Read the model definition and answer for the solid it produces. Units are mm, in the model's axes. A direction names the side the tool comes from. Give positions to 0.01 mm unless a question says otherwise; leave off trailing zeros. Order: outer loops, then holes, each group sorted by start corner. A loop starts at its lowest first (then second) coordinate and runs counter-clockwise, first axis right, second up. Notation, with made-up numbers: (-28.5, 89.5) - (-3.5, 89.5) arc R34 ccw to (-3.5, 122.5) - close; hole circle Ø1 at (86, -17.5). An arc over 180 degrees is marked (long way). Write each question's results on one line, items separated by ' | '.
Autodesk Inventor part; units mm, degrees
ref_plane "YZ Plane" through (0, 0, 0) normal (1, 0, 0) x (0, 1, 0)
ref_plane "XZ Plane" through (0, 0, 0) normal (0, 1, 0) x (-1, 0, 0)
ref_plane "XY Plane" through (0, 0, 0) normal (0, 0, 1) x (1, 0, 0)
sketch "Sketch2" plane through (0, 0, 0) normal (0, 0, 1) x (1, 0, 0)
  line L0 (0, 4) -> (0.5, 4.5)
  line L1 (0, 4) -> (0, 3)
  line L2 (0.5, 4.5) -> (1.1, 4.5)
  line L3 (1.1, 4.5) -> (1.1, 4.3)
  line L4 (1.1, 4.3) -> (2.1, 4.3)
  line L5 (2.1, 4.3) -> (2.1, 4.5)
  line L6 (2.1, 4.5) -> (14.8, 4.5)
  line L7 (15.1, 4.5) -> (15.1, 5.5)
  line L8 (15.1, 5.5) -> (15.6, 6)
  line L9 (44.15, 4.5) -> (44.15, 4.3)
  line L10 (44.15, 4.3) -> (43.15, 4.3)
  line L11 (43.15, 4.3) -> (43.15, 4.5)
  line L12 (0, 0) -> (27.0854, 0) construction
  line L13 (15.6, 6) -> (16.1, 6)
  line L14 (16.1, 6) -> (16.1, 5)
  line L15 (16.1, 5) -> (17.1, 5)
  line L16 (17.1, 5) -> (17.1, 6)
  line L17 (31.9, 6) -> (31.8, 6)
  line L18 (31.5, 6) -> (31.5, 6.5)
  line L19 (31.5, 6.5) -> (28.1, 6.5)
  line L20 (28.1, 6.5) -> (28.1, 6)
  line L21 (17.1, 6) -> (28.1, 6)
  line L22 (21, 3.2) -> (43.9, 3.2)
  line L23 (44.15, 4.5) -> (45.15, 4.5)
  line L24 (43.15, 4.5) -> (37.9, 4.5)
  line L25 (37.15, 6) -> (31.9, 6)
  line L26 (43.9, 3.2) -> (49.9, 3.2)
  line L27 (49.9, 4) -> (45.45, 4)
  line L28 (45.15, 4) -> (45.15, 4.5)
  line L29 (49.9, 3.2) -> (51.9, 3.2)
  line L30 (51.9, 3.2) -> (51.9, 4)
  line L31 (51.9, 4) -> (49.9, 4)
  line L32 (37.9, 4.5) -> (37.45, 4.5)
  line L33 (37.15, 4.5) -> (37.15, 6)
  line L34 (15.1, 4.5) -> (15.1, 4.3)
  line L35 (15.1, 4.3) -> (14.8, 4.3)
  line L36 (14.8, 4.3) -> (14.8, 4.5)
  line L37 (31.5, 6) -> (31.5, 5.8)
  line L38 (31.5, 5.8) -> (31.8, 5.8)
  line L39 (31.8, 5.8) -> (31.8, 6)
  line L40 (37.15, 4.5) -> (37.15, 4.3)
  line L41 (37.15, 4.3) -> (37.45, 4.3)
  line L42 (37.45, 4.3) -> (37.45, 4.5)
  line L43 (45.15, 4) -> (45.15, 3.8)
  line L44 (45.15, 3.8) -> (45.45, 3.8)
  line L45 (45.45, 3.8) -> (45.45, 4)
  line L46 (0, 3) -> (0, 0)
  line L47 (0, 0) -> (20, 0)
  line L48 (20, 2.2) -> (20, 0)
  line L49 (20, 2.2) -> (21, 3.2)
  point P0 (1.1, 4.4)
  point P1 (15.85, 6)
  point P2 (16.6, 5)
  dimension "d3" = 4
  dimension "d8" = 1
  dimension "d9" = 0.5
  dimension "d10" = 0.5
  dimension "d11" = 0.2
  dimension "d12" = 1
  dimension "d13" = 13
  dimension "d14" = 1
  dimension "d29" = 0.5
  dimension "d30" = 0.5
  dimension "d36" = 1.1
  dimension "d37" = 4.5
  dimension "d38" = 3
  dimension "d39" = 0.5
  dimension "d40" = 1
  dimension "d41" = 1
  dimension "d60" = 0.4
  dimension "d61" = 0.5
  dimension "d62" = 3.4
  dimension "d63" = 11
  dimension "d65" = 1
  dimension "d66" = 5.25
  dimension "d83" = 6
  dimension "d84" = 0.8
  dimension "d85" = 2
  dimension "d86" = 0.75
  dimension "d105" = 0.2
  dimension "d106" = 0.3
  dimension "d107" = 0.2
  dimension "d108" = 0.3
  dimension "d109" = 0.2
  dimension "d110" = 0.3
  dimension "d111" = 0.2
  dimension "d112" = 0.3
revolve "Revolution1" add sketch "Sketch2" angle 360 about axis through (0, 0, 0) along (1, 0, 0)
thread "Thread1"
ref_plane "Work Plane1" through (51.1424, -20, -139.2633) normal (0, 1, 0) x (-1, 0, 0)
sketch "Sketch4" plane through (17.1, 0, 0) normal (-1, 0, 0) x (0, 0, 1)
  circle A0 centre (0, 0) radius 6
  point P0 (0, 6)
  point P1 (6, 0)
  point P2 (0, -6.0107)
  point P3 (-6.0435, 0)
chamfer "Chamfer3" distance 0.3 angle 45 1 edges at (51.9, -4, 0)
ref_plane "Work Plane4" through (17.1, 0, 6) normal (0, 0, 1) x (1, 0, 0)
sketch "Sketch8" plane through (17.1, 0, 6) normal (0, 0, 1) x (1, 0, 0)
  circle A0 centre (6.1, 0) radius 1
  line L0 (0, -6) -> (0, 6)
  point P0 (-17.1, 0)
  dimension "d90" = 2
  dimension "d91" = 6.1
hole "Hole3" at (23.2, 0, 6) direction (0, 0, -1) diameter 1.567 depth 6.3 tip angle 118
chamfer "Chamfer4" distance 0.2 angle 45 3 edges at (22.6668, -0.5741, 5.9725) (23.7332, -0.5741, 5.9725) (23.2, 0.7835, 5.9486)
chamfer "Chamfer5" distance 0.3 angle 45 1 edges at (51.9, -3.2, 0)
sketch "Sketch9" plane through (0, 0, 0) normal (-1, 0, 0) x (0, 0, 1)
  circle A0 centre (0, 0) radius 1.2953
hole "Hole4" at (0, 0, 0) direction (1, 0, 0) diameter 4.917 end through all
chamfer "Chamfer6" distance 0.5 angle 45 1 edges at (0, 0, -2.4585)
properties part number "nakrętka otwor w pionie"
(1) Section B-B (y = 0) is taken. State how many separate pieces and enclosed holes the cut face has, plus the area to 3 significant figures.
Conclusion:
separate pieces: 3 | enclosed holes: 0 | area: 220 mm^2
(2) For faces 4 (the face through (48.482, -0.867, 3.905)), 5 (the face through (22.54, -0.42, 4.43)), 6 (the face through (0.8, -0.59, 4.46)), 7 (the face through (31.5, -6, 0)), determine the directions among +Z, -Z, +X, -X, +Y, -Y from which every point of the face is accessible in a straight line to the end or side of a thin tool.
Conclusion:
face 4: +X | face 5: +Z | face 6: -X | face 7: none
(3) Each of these flat-tipped pins is pushed along its axis until it touches: pin 1 (1.4 mm diameter, centred on x = 23.2, y = 0, fed in from +Z); pin 2 (3 mm diameter, centred on x = 32.5, y = 4, fed in from +Z); pin 3 (2 mm diameter, centred on x = 32, z = -3.5, fed in from +Y). Where does it stop, or does it pass through?
Conclusion:
pin 1: z = -3.12 | pin 2: z = 5.83 | pin 3: y = 5.94
(4) Section C-C (x = 4) is taken. Give the vertices of the cut face in (y, z).
Conclusion:
outline: circle Ø9 at (0, 0); hole circle Ø4.92 at (0, 0)
(5) The mould has two halves that part along X. Classify faces 1 (the face through (31.65, -4.6, -3.53)), 2 (the face through (28.1, 2, -6)), 3 (the face through (29.776, -5.158, 3.955)): pulls with the +X half, pulls with the -X half, needs draft (parallel to the pull), parting line crosses it, or undercut.
Conclusion:
face 1: undercut | face 2: pulls with the -X half | face 3: needs draft
(6) Consider probe 1 along X at (y, z) = (-2, -4.75); probe 2 along Z at (x, y) = (8.5, 0); probe 3 along Y at (x, z) = (14.5, -0.5). Determine where each line is inside the solid, lowest interval first. Write a range as [from, to].
Conclusion:
probe 1: [15.1, 16.1], [17.1, 37.15] | probe 2: [-4.5, -2.46], [2.46, 4.5] | probe 3: [-4.47, -2.41], [2.41, 4.47]
(7) Section A-A (x = 31) is taken. Give the vertices of the cut face in (y, z), plus the area to 3 significant figures.
Conclusion:
outline: circle Ø13 at (0, 0); hole circle Ø6.4 at (0, 0) | area: 101 mm^2
